Read the model definition and answer for the solid it produces. Units are mm, in the model's axes. Round coordinates to 2 decimals unless told otherwise and drop trailing zeros. Order: outer loops, then holes, each group sorted by start corner. A loop starts at its lowest first (then second) coordinate and runs counter-clockwise, first axis right, second up. Notation, with made-up numbers: (34, 19) -> (38, 19) arc R29 ccw to (38, 42) -> close; hole circle Ø6 at (86, 78). An arc over 180 degrees is marked (long way). Use a Markdown table: item, result. Add a question column.
1. Section A-A, the plane z = -29.5 is taken. Give the vertices of the cut face in (x, y) (3 decimals).
2. Given pin 1 (1.5 mm diameter, centred on x = 23, y = -0.5, fed in from +Z), flat-ended and moving along its own axis, determine where the tip first touches the part or whether it passes through.
3. Consider L1, parallel to Z at x = 54, y = -0.7; L2, parallel to X at y = -1.95, z = 66; L3, parallel to Z at x = 32, y = -1. Determine where each line is inside the solid, lowest interval first. Write a range as [from, to].
```python
from build123d import *

# Parameters (mm, degrees)
F2_DEPTH = 3.175
F3_D     = 12.7


with BuildPart() as f2:
    # F0 (on Front) → F2 (new body)
    with BuildSketch(Plane.XZ):
        with BuildLine():
            ThreePointArc((5.7552136035, 75.9823500319), (3.3237973172, 76.1274744845), (0.8889848745, 76.1948141667))
            ThreePointArc((0.8889848745, 76.1948141667), (0.6267817779, 75.5695512686), (0, 75.311))
            Line((0, 75.311), (0, -75.311))
            ThreePointArc((0, -75.311), (0.6267817779, -75.5695512686), (0.8889848745, -76.1948141667))
            ThreePointArc((0.8889848745, -76.1948141667), (3.3237973172, -76.1274744845), (5.7552136035, -75.9823500319))
            ThreePointArc((5.7552136035, -75.9823500319), (6.5637861421, -75.024418908), (7.5264176409, -75.8273897579))
            ThreePointArc((7.5264176409, -75.8273897579), (9.9460958472, -75.5480984367), (12.355611431, -75.1916143341))
            ThreePointArc((12.355611431, -75.1916143341), (13.0776179083, -74.1668566871), (14.1065698245, -74.8828731272))
            ThreePointArc((14.1065698245, -74.8828731272), (16.4926985821, -74.3937557425), (18.8619755949, -73.8286250492))
            ThreePointArc((18.8619755949, -73.8286250492), (19.4919211057, -72.7448399037), (20.5793624939, -73.3684526165))
            ThreePointArc((20.5793624939, -73.3684526165), (22.9137819222, -72.673231647), (25.2247887354, -71.9037553488))
            ThreePointArc((25.2247887354, -71.9037553488), (25.757879014, -70.769190964), (26.8955337885, -71.2956538804))
            ThreePointArc((26.8955337885, -71.2956538804), (29.1604775462, -70.3996203774), (31.3956260024, -69.4316546534))
            ThreePointArc((31.3956260024, -69.4316546534), (31.82780391, -68.2549457495), (33.0070138311, -68.6802521687))
            ThreePointArc((33.0070138311, -68.6802521687), (35.1852443285, -67.5902254882), (37.3275235984, -66.4311371422))
            ThreePointArc((37.3275235984, -66.4311371422), (37.6555, -65.2212391844), (38.8672905683, -65.5421522677))
            ThreePointArc((38.8672905683, -65.5421522677), (40.942230156, -64.2664281709), (42.9753362008, -62.9250385651))
            ThreePointArc((42.9753362008, -62.9250385651), (43.196614998, -61.6911596074), (44.4317637555, -61.9052370125))
            ThreePointArc((44.4317637555, -61.9052370125), (46.3876208905, -60.4535245302), (48.2960805456, -58.9400424494))
            ThreePointArc((48.2960805456, -58.9400424494), (48.4089776731, -57.6915730557), (49.6580843918, -57.7971855243))
            ThreePointArc((49.6580843918, -57.7971855243), (51.4799738203, -56.1805330649), (53.2492625554, -54.5064770216))
            ThreePointArc((53.2492625554, -54.5064770216), (53.2529187979, -53.2529187979), (54.5064770216, -53.2492625554))
            ThreePointArc((54.5064770216, -53.2492625554), (56.1805330649, -51.4799738203), (57.7971855243, -49.6580843918))
            ThreePointArc((57.7971855243, -49.6580843918), (57.6915730557, -48.4089776731), (58.9400424494, -48.2960805456))
            ThreePointArc((58.9400424494, -48.2960805456), (60.4535245302, -46.3876208905), (61.9052370125, -44.4317637555))
            ThreePointArc((61.9052370125, -44.4317637555), (61.6911596074, -43.196614998), (62.9250385651, -42.9753362008))
            ThreePointArc((62.9250385651, -42.9753362008), (64.2664281709, -40.942230156), (65.5421522677, -38.8672905683))
            ThreePointArc((65.5421522677, -38.8672905683), (65.2212391844, -37.6555), (66.4311371422, -37.3275235984))
            ThreePointArc((66.4311371422, -37.3275235984), (67.5902254882, -35.1852443285), (68.6802521687, -33.0070138311))
            ThreePointArc((68.6802521687, -33.0070138311), (68.2549457495, -31.82780391), (69.4316546534, -31.3956260024))
            ThreePointArc((69.4316546534, -31.3956260024), (70.3996203774, -29.1604775462), (71.2956538804, -26.8955337885))
            ThreePointArc((71.2956538804, -26.8955337885), (70.769190964, -25.757879014), (71.9037553488, -25.2247887354))
            ThreePointArc((71.9037553488, -25.2247887354), (72.673231647, -22.9137819222), (73.3684526165, -20.5793624939))
            ThreePointArc((73.3684526165, -20.5793624939), (72.7448399037, -19.4919211057), (73.8286250492, -18.8619755949))
            ThreePointArc((73.8286250492, -18.8619755949), (74.3937557425, -16.4926985821), (74.8828731272, -14.1065698245))
            ThreePointArc((74.8828731272, -14.1065698245), (74.1668566871, -13.0776179083), (75.1916143341, -12.355611431))
            ThreePointArc((75.1916143341, -12.355611431), (75.5480984367, -9.9460958472), (75.8273897579, -7.5264176409))
            ThreePointArc((75.8273897579, -7.5264176409), (75.024418908, -6.5637861421), (75.9823500319, -5.7552136035))
            ThreePointArc((75.9823500319, -5.7552136035), (76.1274744845, -3.3237973172), (76.1948141667, -0.8889848745))
            ThreePointArc((76.1948141667, -0.8889848745), (75.311, 0), (76.1948141667, 0.8889848745))
            ThreePointArc((76.1948141667, 0.8889848745), (76.1274744845, 3.3237973172), (75.9823500319, 5.7552136035))
            ThreePointArc((75.9823500319, 5.7552136035), (75.024418908, 6.5637861421), (75.8273897579, 7.5264176409))
            ThreePointArc((75.8273897579, 7.5264176409), (75.5480984367, 9.9460958472), (75.1916143341, 12.355611431))
            ThreePointArc((75.1916143341, 12.355611431), (74.1668566871, 13.0776179083), (74.8828731272, 14.1065698245))
            ThreePointArc((74.8828731272, 14.1065698245), (74.3937557425, 16.4926985821), (73.8286250492, 18.8619755949))
            ThreePointArc((73.8286250492, 18.8619755949), (72.7448399037, 19.4919211057), (73.3684526165, 20.5793624939))
            ThreePointArc((73.3684526165, 20.5793624939), (72.673231647, 22.9137819222), (71.9037553488, 25.2247887354))
            ThreePointArc((71.9037553488, 25.2247887354), (70.769190964, 25.757879014), (71.2956538804, 26.8955337885))
            ThreePointArc((71.2956538804, 26.8955337885), (70.3996203774, 29.1604775462), (69.4316546534, 31.3956260024))
            ThreePointArc((69.4316546534, 31.3956260024), (68.2549457495, 31.82780391), (68.6802521687, 33.0070138311))
            ThreePointArc((68.6802521687, 33.0070138311), (67.5902254882, 35.1852443285), (66.4311371422, 37.3275235984))
            ThreePointArc((66.4311371422, 37.3275235984), (65.2212391844, 37.6555), (65.5421522677, 38.8672905683))
            ThreePointArc((65.5421522677, 38.8672905683), (64.2664281709, 40.942230156), (62.9250385651, 42.9753362008))
            ThreePointArc((62.9250385651, 42.9753362008), (61.6911596074, 43.196614998), (61.9052370125, 44.4317637555))
            ThreePointArc((61.9052370125, 44.4317637555), (60.4535245302, 46.3876208905), (58.9400424494, 48.2960805456))
            ThreePointArc((58.9400424494, 48.2960805456), (57.6915730557, 48.4089776731), (57.7971855243, 49.6580843918))
            ThreePointArc((57.7971855243, 49.6580843918), (56.1805330649, 51.4799738203), (54.5064770216, 53.2492625554))
            ThreePointArc((54.5064770216, 53.2492625554), (53.2529187979, 53.2529187979), (53.2492625554, 54.5064770216))
            ThreePointArc((53.2492625554, 54.5064770216), (51.4799738203, 56.1805330649), (49.6580843918, 57.7971855243))
            ThreePointArc((49.6580843918, 57.7971855243), (48.4089776731, 57.6915730557), (48.2960805456, 58.9400424494))
            ThreePointArc((48.2960805456, 58.9400424494), (46.3876208905, 60.4535245302), (44.4317637555, 61.9052370125))
            ThreePointArc((44.4317637555, 61.9052370125), (43.196614998, 61.6911596074), (42.9753362008, 62.9250385651))
            ThreePointArc((42.9753362008, 62.9250385651), (40.942230156, 64.2664281709), (38.8672905683, 65.5421522677))
            ThreePointArc((38.8672905683, 65.5421522677), (37.6555, 65.2212391844), (37.3275235984, 66.4311371422))
            ThreePointArc((37.3275235984, 66.4311371422), (35.1852443285, 67.5902254882), (33.0070138311, 68.6802521687))
            ThreePointArc((33.0070138311, 68.6802521687), (31.82780391, 68.2549457495), (31.3956260024, 69.4316546534))
            ThreePointArc((31.3956260024, 69.4316546534), (29.1604775462, 70.3996203774), (26.8955337885, 71.2956538804))
            ThreePointArc((26.8955337885, 71.2956538804), (25.757879014, 70.769190964), (25.2247887354, 71.9037553488))
            ThreePointArc((25.2247887354, 71.9037553488), (22.9137819222, 72.673231647), (20.5793624939, 73.3684526165))
            ThreePointArc((20.5793624939, 73.3684526165), (19.4919211057, 72.7448399037), (18.8619755949, 73.8286250492))
            ThreePointArc((18.8619755949, 73.8286250492), (16.4926985821, 74.3937557425), (14.1065698245, 74.8828731272))
            ThreePointArc((14.1065698245, 74.8828731272), (13.0776179083, 74.1668566871), (12.355611431, 75.1916143341))
            ThreePointArc((12.355611431, 75.1916143341), (9.9460958472, 75.5480984367), (7.5264176409, 75.8273897579))
            ThreePointArc((7.5264176409, 75.8273897579), (6.5637861421, 75.024418908), (5.7552136035, 75.9823500319))
        make_face()
    extrude(amount=F2_DEPTH)

    # F3 (through all)
    with Locations(Plane(origin=(0, 0, 0), x_dir=(1, 0, 0), z_dir=(0, 1, 0))):
        with Locations((0, 0)):
            Hole(F3_D / 2)


solid = f2.part
```
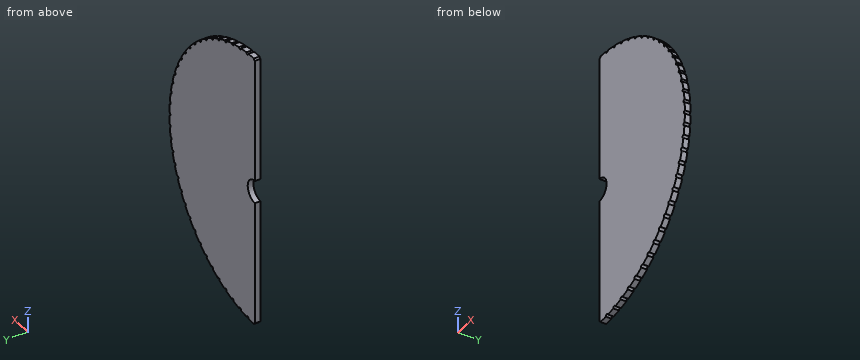
Verdict:
| question | item | result |
|---|---|---|
| 1 | outline | (0, -3.175) -> (70.258, -3.175) -> (70.258, 0) -> (0, 0) -> close |
| 2 | pin 1 | stops at z = 72.88 |
| 3 | L1 | z = [-53, 53] |
| 3 | L2 | x = [0, 37.21] |
| 3 | L3 | z = [-68.2, 68.2] |
